Answer from the drawing. Dimensions are ordinates in mm from the lowest x, y and z of the part. Give positions to 0.01 mm unless a question says otherwise; leave off trailing zeros. Order: outer loops, then holes, each group sorted by start corner. A loop starts at its lowest first (then second) coordinate and runs counter-clockwise, first axis right, second up. Notation, with made-up numbers: (88, 73.25) - (116, 73.25) arc R35 cw to (116, 111.25) - close; hole circle Ø7 at (-5.75, 10.5). An arc over 180 degrees is marked (long way). Use a Markdown table: item, result. Add a question column.
1) The mould has two halves that part along X. Classify the marked faces 1, 2, 3 and 4: released by +X, released by -X, zero draft, split by the parting line, or undercut.
2) Find section C-C, the plane x = 4.5. Determine the outline of the cut face in (y, z), plus the area to 3 significant figures.
3) Find section A-A, the plane z = 11.6. Determine the outline of the cut face in (x, y).
4) Find section B-B, the plane y = 0.95. Determine the outline of the cut face in (x, z).
5) Straight lines are drawn through the part: line 1 (Z direction, x = 3.2, y = 3.1); line 2 (X direction, y = 0.9, z = 4.5); line 3 (Z direction, x = 14.6, y = 3.8). For each, find the intervals that lie inside material, in ascending order.
6) A flat-ended cylindrical pin translates along its axis: pin 1 (3 mm diameter, centred on y = 1.5, z = 12.5, fed in from -X). Find the tip coordinate at first contact, or state that the pin passes through.
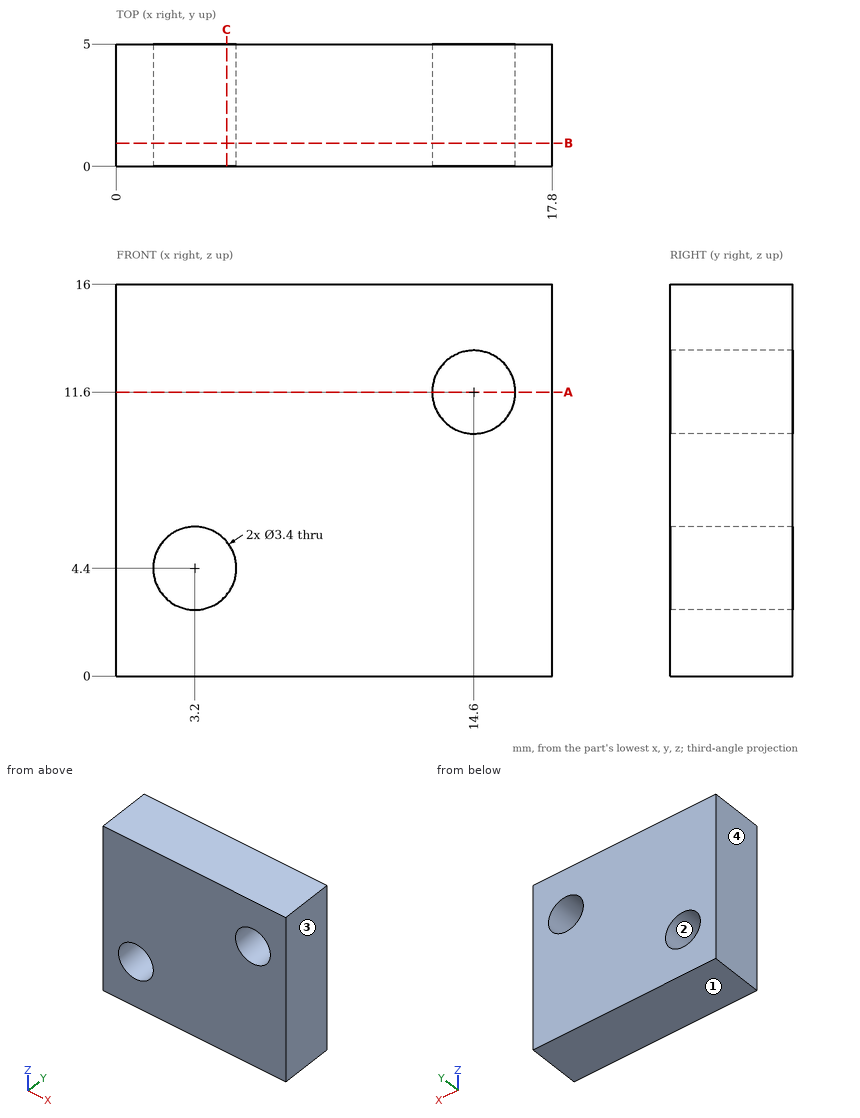
The answers:
| question | item | result |
|---|---|---|
| 1 | face 1 | zero draft |
| 1 | face 2 | undercut |
| 1 | face 3 | released by +X |
| 1 | face 4 | released by -X |
| 2 | outline | (0, 0) - (5, 0) - (5, 3.3) - (0, 3.3) - close; (0, 5.5) - (5, 5.5) - (5, 16) - (0, 16) - close |
| 2 | area | 69.0 mm2 |
| 3 | outline | (0, 0) - (12.9, 0) - (12.9, 5) - (0, 5) - close; (16.3, 0) - (17.8, 0) - (17.8, 5) - (16.3, 5) - close |
| 4 | outline | (0, 0) - (17.8, 0) - (17.8, 16) - (0, 16) - close; hole circle Ø3.4 at (3.2, 4.4); hole circle Ø3.4 at (14.6, 11.6) |
| 5 | line 1 | 0 to 2.7, 6.1 to 16 |
| 5 | line 2 | 0 to 1.5, 4.9 to 17.8 |
| 5 | line 3 | 0 to 9.9, 13.3 to 16 |
| 6 | pin 1 | x = 0 |
